Work out the finished part from the listing and answer in its coordinate system (mm). Face numbers are marked on the shaded views. Give positions to 0.01 mm unless a question says otherwise; leave off trailing zeros. Write each loop counter-clockwise with the first axis right and the second up, starting at its lowest first coordinate (ties: lowest second). Pieces come first, ordered by that corner, then holes. Notation, with made-up numbers: (20, -9.5) -> (50, -9.5) arc R25 ccw to (50, 13.5) -> close; hole circle Ø11 at (-19, 48). An arc over 180 degrees is marked (long way). Write item = value, one per line. Start each with the question number.
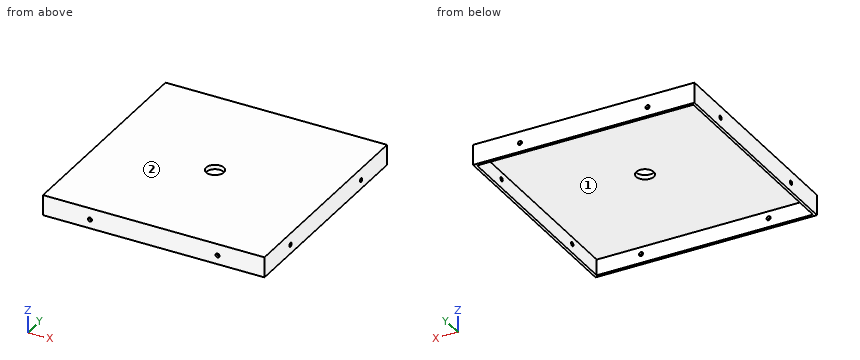
from build123d import *

# Parameters (mm, degrees)
SKETCH_1_W               = 250
SKETCH_1_H               = 250
SKETCH_1_R               = 10
EXTRUDE_1_DEPTH          = 5
SKETCH_3_W               = 250
SKETCH_3_H               = 250
SKETCH_3_W_2             = 244
SKETCH_3_H_2             = 244
EXTRUDE_2_DEPTH          = 18
HOLE_WIZARD_M4_1_D       = 4.6
HOLE_WIZARD_M4_1_DEPTH   = 3
PATTERN_CIRCULAR_1_COUNT = 4


with BuildPart() as part:
    # 스케치1 → 보스-돌출1 (new body)
    with BuildSketch(Plane.XY):
        Rectangle(SKETCH_1_W, SKETCH_1_H)
        Circle(SKETCH_1_R, mode=Mode.SUBTRACT)
    extrude(amount=EXTRUDE_1_DEPTH)

    # 스케치3 → 보스-돌출2 (add)
    with BuildSketch(Plane(origin=(0, 0, 0), x_dir=(-1, 0, 0), z_dir=(0, 0, -1))):
        Rectangle(SKETCH_3_W, SKETCH_3_H)
        Rectangle(SKETCH_3_W_2, SKETCH_3_H_2, mode=Mode.SUBTRACT)
    extrude(amount=EXTRUDE_2_DEPTH)

    # M4 여유 구멍1
    with Locations(Plane.ZY.offset(-122)):
        with Locations((-8, 72), (-8, -72)):
            hole_wizard_m4_1 = Hole(HOLE_WIZARD_M4_1_D / 2, depth=HOLE_WIZARD_M4_1_DEPTH)

    # 원형 패턴1: M4 여유 구멍1 ×4 about axis
    pattern_circular_1_axis = Axis((0, 0, 0), (0, 0, 1))
    for i in range(1, PATTERN_CIRCULAR_1_COUNT):
        add(hole_wizard_m4_1.rotate(pattern_circular_1_axis, i * 360 / PATTERN_CIRCULAR_1_COUNT), mode=Mode.SUBTRACT)


solid = part.part
(1) A cutting plane is placed at A-A, the plane y = 0. Write down the section's boundary in (x, z).
(2) This flat-tipped pin is pushed along its axis until it touches: pin 1 (1 mm diameter, centred on x = -27.5, y = -97, fed in from -Z). Where does it stop, or does it pass through?
(3) Determine the mould class of the marked faces 1 and 2 for opening direction X: pulls with the +X half, pulls with the -X half, needs draft (parallel to the pull), parting line crosses it, or undercut.
(4) Find the intervals of material crossed by line 1 along X through (y, z) = (97, -7); line 2 along Z through (x, y) = (-72, -123.3), in increasing order.
(5) A cutting plane is placed at C-C, the plane x = -95.5. Write down the section's boundary in (y, z).
Results list:
q1.outline = (-125, -18) -> (-122, -18) -> (-122, 0) -> (-10, 0) -> (-10, 5) -> (-125, 5) -> close; (10, 0) -> (122, 0) -> (122, -18) -> (125, -18) -> (125, 5) -> (10, 5) -> close
q2.pin_1 = 0
q3.face_1 = undercut
q3.face_2 = needs draft
q4.line_1 = -125 to -122, 122 to 125
q4.line_2 = -18 to -10.3, -5.7 to 5
q5.outline = (-125, -18) -> (-122, -18) -> (-122, 0) -> (122, 0) -> (122, -18) -> (125, -18) -> (125, 5) -> (-125, 5) -> close
